Verification items for the finished model (mm, model axes). A direction names the side the tool comes from. Round coordinates to 2 decimals unless told otherwise and drop trailing zeros. Loops run counter-clockwise (first coordinate to the right, second up) from the corner with the lowest first, then second, coordinate; pieces in that order, holes last.
from build123d import *

# Parameters (mm, degrees)
BOSS_EXTRUDE1_DEPTH   = 76.2
F_8_CLEARANCE_HOLE1_D = 4.4958
F_8_CLEARANCE_HOLE2_D = 4.4958


with BuildPart() as part:
    # Sketch1 → Boss-Extrude1 (new body)
    with BuildSketch(Plane.XY):
        Polygon((0, 0), (25.4, 0), (25.4, 3.175), (3.175, 3.175), (3.175, 25.4), (0, 25.4), align=None)
    extrude(amount=BOSS_EXTRUDE1_DEPTH)

    # #8 Clearance Hole1 (through all)
    with Locations(Plane.XZ):
        with Locations((12.7, 63.5), (12.7, 38.1), (12.7, 12.7)):
            Hole(F_8_CLEARANCE_HOLE1_D / 2)

    # #8 Clearance Hole2 (through all)
    with Locations(Plane.ZY):
        with Locations((63.5, 12.7), (38.1, 12.7), (12.7, 12.7)):
            Hole(F_8_CLEARANCE_HOLE2_D / 2)


solid = part.part
1. Scan lines: L1, parallel to Z at x = 12.7, y = 1.6; L2, parallel to Y at x = 1.05, z = 63.5; L3, parallel to X at y = 17.5, z = 54 (3 decimals). Record each from-to range of solid material in increasing order.
2. Section check B-B (z = 63.5). Enter the section's corners in (x, y) (3 decimals).
3. Section check D-D (x = 9.5). Enter the section's corners in (y, z) (3 decimals).
4. Section check A-A (x = 12.7). Enter the section's corners in (y, z) (3 decimals), then the cut area to 3 significant figures.
5. Tool access check on faces 1 (the face through (1.61, 12.799, 65.746)), 2 (the face through (17, 3.175, 38)). Record the directions out of +Z, -Z, +X, -X, +Y, -Y that give a thin tool (end or side, any length) a straight path to the whole face; none if there is none.
6. Release check for a two-part mould opening along X. For faces 3 (the face through (0, 10, 38)), 4 (the face through (3.175, 17, 38)), 5 (the face through (1.61, 14.219, 14.357)), 6 (the face through (12.99, 1.61, 40.33)) record: released by +X, released by -X, zero draft, split by the parting line, or undercut.
7. Gauge pin test, flat ends, axial feed: P1, Ø1, axis at x = 16.5, z = 42, coming from the +Y side (3 decimals); P2, Ø4, axis at y = 12.7, z = 38.1, coming from the -X side; P3, Ø2, axis at y = 15.5, z = 21, coming from the +X side (3 decimals). Record the tip position at first contact, or that the pin passes through.
Taken from the geometry:
1. L1: z = 0 to 10.45, 14.95 to 35.85, 40.35 to 61.25, 65.75 to 76.2
1. L2: y = 0 to 10.45, 14.95 to 25.4
1. L3: x = 0 to 3.175
2. outline: (0, 0) - (10.452, 0) - (10.452, 3.175) - (3.175, 3.175) - (3.175, 10.452) - (0, 10.452) - close; (0, 14.948) - (3.175, 14.948) - (3.175, 25.4) - (0, 25.4) - close; (14.948, 0) - (25.4, 0) - (25.4, 3.175) - (14.948, 3.175) - close
3. outline: (0, 0) - (3.175, 0) - (3.175, 76.2) - (0, 76.2) - close
4. outline: (0, 0) - (3.175, 0) - (3.175, 10.452) - (0, 10.452) - close; (0, 14.948) - (3.175, 14.948) - (3.175, 35.852) - (0, 35.852) - close; (0, 40.348) - (3.175, 40.348) - (3.175, 61.252) - (0, 61.252) - close; (0, 65.748) - (3.175, 65.748) - (3.175, 76.2) - (0, 76.2) - close
4. area: 199 mm2
5. face 1: +X, -X
5. face 2: +Z, -Z, +X, +Y
6. face 3: released by -X
6. face 4: released by +X
6. face 5: zero draft
6. face 6: undercut
7. P1: stops at y = 3.175
7. P2: passes through
7. P3: stops at x = 3.175
